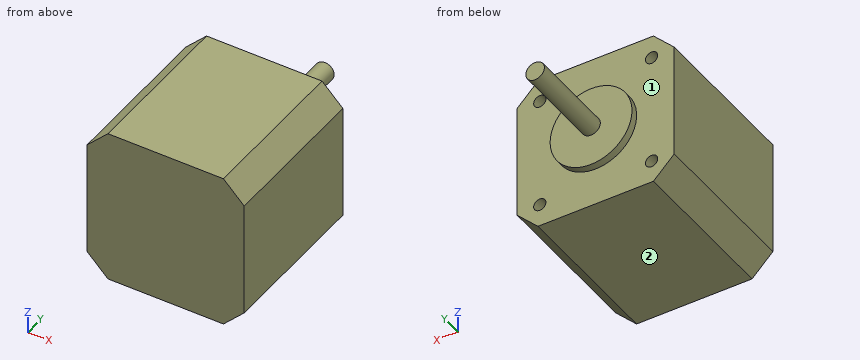
```python
from build123d import *

# Parameters (mm, degrees)
ESBO_O1_W                = 42.3
ESBO_O1_H                = 42.3
RESSALTO_EXTRUS_O1_DEPTH = 21.15
ESBO_O2_R                = 11.025
RESSALTO_EXTRUS_O2_DEPTH = 2
ESBO_O3_R                = 2.506
RESSALTO_EXTRUS_O3_DEPTH = 24
CHANFRO1_SIZE            = 5.6
ESBO_O4_R                = 1.65
CORTE_EXTRUS_O1_DEPTH    = 10


with BuildPart() as part:
    # Esboço1 → Ressalto-extrusão1 (new body, symmetric)
    with BuildSketch(Plane(origin=(0, 0, 0), x_dir=(1, 0, 0), z_dir=(0, 1, 0))):
        Rectangle(ESBO_O1_W, ESBO_O1_H)
    extrude(amount=RESSALTO_EXTRUS_O1_DEPTH, both=True)

    # Esboço2 → Ressalto-extrusão2 (add)
    with BuildSketch(Plane(origin=(0, 21.15, 0), x_dir=(1, 0, 0), z_dir=(0, 1, 0))):
        Circle(ESBO_O2_R)
    extrude(amount=RESSALTO_EXTRUS_O2_DEPTH)

    # Esboço3 → Ressalto-extrusão3 (add)
    with BuildSketch(Plane(origin=(0, 23.15, 0), x_dir=(1, 0, 0), z_dir=(0, 1, 0))):
        Circle(ESBO_O3_R)
    extrude(amount=RESSALTO_EXTRUS_O3_DEPTH)

    # Chanfro1
    chanfro1_edges = [part.edges().sort_by_distance(p)[0] for p in [
        (21.15, 0, 21.15),
        (-21.15, 0, 21.15),
        (-21.15, 0, -21.15),
        (21.15, 0, -21.15),
    ]]
    chamfer(chanfro1_edges, length=CHANFRO1_SIZE)

    # Esboço4 → Corte-extrusão1 (cut)
    with BuildSketch(Plane(origin=(0, 21.15, 0), x_dir=(1, 0, 0), z_dir=(0, 1, 0))):
        with Locations((-15.05, 15.05)):
            Circle(ESBO_O4_R)
        with Locations((15.05, 15.05)):
            Circle(ESBO_O4_R)
        with Locations((15.05, -15.05)):
            Circle(ESBO_O4_R)
        with Locations((-15.05, -15.05)):
            Circle(ESBO_O4_R)
    extrude(amount=-CORTE_EXTRUS_O1_DEPTH, mode=Mode.SUBTRACT)


solid = part.part
```
Verification items for the finished model (mm, model axes). Face numbers are marked on the shaded views. A direction names the side the tool comes from. Give positions to 0.01 mm unless a question says otherwise; leave off trailing zeros. Order: outer loops, then holes, each group sorted by start corner. A loop starts at its lowest first (then second) coordinate and runs counter-clockwise, first axis right, second up. Notation, with made-up numbers: M 1,27.5 L 30,27.5 A16 ccw 30,47.5 Z; hole C 60,89.25 d8. An arc over 180 degrees is marked long. Answer in a Markdown table with one row per item. Add a question column.
Item 1: Section check D-D, the plane x = -18. Enter the section's corners in (y, z), and give its area (3 significant figures).
Item 2: Scan lines: probe 1 along X at (y, z) = (16.5, -15.05); probe 2 along Y at (x, z) = (-1.5, 10). Record each from-to range of solid material in increasing order. Write a range as from..to.
Item 3: Section check A-A, the plane x = 0. Enter the section's corners in (y, z) (3 decimals).
Item 4: Section check C-C, the plane z = 9. Enter the section's corners in (x, y).
Item 5: Tool access check on the marked faces 1 and 2. Record the directions out of +Z, -Z, +X, -X, +Y, -Y that give a thin tool (end or side, any length) a straight path to the whole face; none if there is none.
Item 6: Section check B-B, the plane y = -4. Enter the section's corners in (x, z).
Item 7: Gauge pin test, flat ends, axial feed: pin 1 (1 mm diameter, centred on x = 14.5, z = 15, fed in from +Y); pin 2 (4 mm diameter, centred on x = 12, z = 12, fed in from +Y); pin 3 (12 mm diameter, centred on x = 0, z = 14, fed in from +Y). Record the tip position at first contact, or that the pin passes through.
Filled sheet:
| question | item | result |
|---|---|---|
| 1 | outline | M -21.15,-18.7 L 21.15,-18.7 L 21.15,18.7 L -21.15,18.7 Z |
| 1 | area | 1,580 mm^2 |
| 2 | probe 1 | x = -21.15..-16.7, -13.4..13.4, 16.7..21.15 |
| 2 | probe 2 | y = -21.15..23.15 |
| 3 | outline | M -21.15,-21.15 L 21.15,-21.15 L 21.15,-11.025 L 23.15,-11.025 L 23.15,-2.506 L 47.15,-2.506 L 47.15,2.506 L 23.15,2.506 L 23.15,11.025 L 21.15,11.025 L 21.15,21.15 L -21.15,21.15 Z |
| 4 | outline | M -21.15,-21.15 L 21.15,-21.15 L 21.15,21.15 L 6.37,21.15 L 6.37,23.15 L -6.37,23.15 L -6.37,21.15 L -21.15,21.15 Z |
| 5 | face 1 | +Y |
| 5 | face 2 | -Z, +X, -X, +Y, -Y |
| 6 | outline | M -21.15,-15.55 L -15.55,-21.15 L 15.55,-21.15 L 21.15,-15.55 L 21.15,15.55 L 15.55,21.15 L -15.55,21.15 L -21.15,15.55 Z |
| 7 | pin 1 | stops at y = 11.15 |
| 7 | pin 2 | stops at y = 21.15 |
| 7 | pin 3 | stops at y = 23.15 |
